from build123d import *

# Parameters (mm, degrees)
BLANKSKE_W        = 50
BLANKSKE_H        = 5.7
BLANK_DEPTH       = 6
TOOTHCUTSIM_DEPTH = 51.680272296
TEETHCUTS_COUNT   = 24
TEETHCUTS_PITCH   = 2.199114855
SKETCH_1_W        = 6
SKETCH_1_H        = 4.125
EXTRUDE_1_DEPTH   = 47


with BuildPart() as part:
    # BlankSke → Blank (new body)
    with BuildSketch(Plane.XY):
        with Locations((25, 2.85)):
            Rectangle(BLANKSKE_W, BLANKSKE_H)
    extrude(amount=-BLANK_DEPTH)

    # TooCutSkeSim → ToothCutSim (cut, through all)
    with BuildSketch(Plane.XY):
        Polygon((0.312304759, 4.125), (-0.312304759, 4.125), (-0.894802722, 5.7254), (0.894802722, 5.7254), align=None)
    toothcutsim = extrude(amount=-TOOTHCUTSIM_DEPTH, mode=Mode.SUBTRACT)

    # TeethCuts: ToothCutSim ×24
    with Locations(*[(i * TEETHCUTS_PITCH, 0, 0) for i in range(1, TEETHCUTS_COUNT)]):
        add(toothcutsim, mode=Mode.SUBTRACT)

    # 草图1 → 凸台-拉伸1 (add)
    with BuildSketch(Plane.ZY):
        with Locations((-3, 2.0625)):
            Rectangle(SKETCH_1_W, SKETCH_1_H)
    extrude(amount=EXTRUDE_1_DEPTH)


solid = part.part
The listing builds one solid part. Answer for the finished solid, in the listing's coordinates (mm). A direction names the side the tool comes from. Coordinates: 2 decimals unless noted, no trailing zeros. Write each loop counter-clockwise with the first axis right and the second up, starting at its lowest first coordinate (ties: lowest second). Pieces come first, ordered by that corner, then holes. Notation, with made-up numbers: (-17, 81) - (31, 81) arc R8 ccw to (31, 91) - close; hole circle Ø1 at (66, 30.5). An arc over 180 degrees is marked (long way). Put each result on its own line as item: value.
1. Determine the mould class of faces 1 (the face through (-47, 2, -3)), 2 (the face through (34.59, 4.9, -2.96)), 3 (the face through (50, 2, -3)), 4 (the face through (2, 2, -6)) for opening direction X: pulls with the +X half, pulls with the -X half, needs draft (parallel to the pull), parting line crosses it, or undercut.
Answer sheet:
face 1: pulls with the -X half
face 2: undercut
face 3: pulls with the +X half
face 4: needs draft
2. Find the intervals of material crossed by line 1 along Y through (x, z) = (-7.5, -4.5) (3 decimals), in increasing order. Write a range as from..to.
Answer sheet:
line 1: y = 0..4.125
3. A flat-ended cylindrical pin translates along its axis: pin 1 Ø1.5 at (x, y) = (30.5, 4.5) entering from +Z. Find the tip coordinate at first contact, or state that the pin passes through.
Answer sheet:
pin 1: stops at z = 0
4. The part is cut by section A-A on x = -18. Give the vertices of the cut face in (y, z) (3 decimals).
Answer sheet:
outline: (0, -6) - (4.125, -6) - (4.125, 0) - (0, 0) - close
5. A tool of negligible diameter and unlimited length cuts with its end or side. For faces 5 (the face through (2, 0, -3)), 6 (the face through (15.997, 4.924, -2.958)), from which of +Z, -Z, +X, -X, +Y, -Y can it reach the whole face along a straight path? Write none if from no direction.
Answer sheet:
face 5: +Z, -Z, +X, -X, -Y
face 6: +Z, -Z, +Y
